The figure shows three views and two pictorial views of one solid part (mm, origin at its lowest corner). Answer the questions. A direction names the side the tool comes from. Coordinates: 2 decimals unless noted, no trailing zeros. Loops run counter-clockwise (first coordinate to the right, second up) from the corner with the lowest first, then second, coordinate; pieces in that order, holes last. Notation, with made-up numbers: (7.25, 82) -> (17.25, 82) arc R30 cw to (17.25, 110) -> close; hole circle Ø1 at (38, 68). An arc over 180 degrees is marked (long way). Answer in a Markdown table with one row per item.
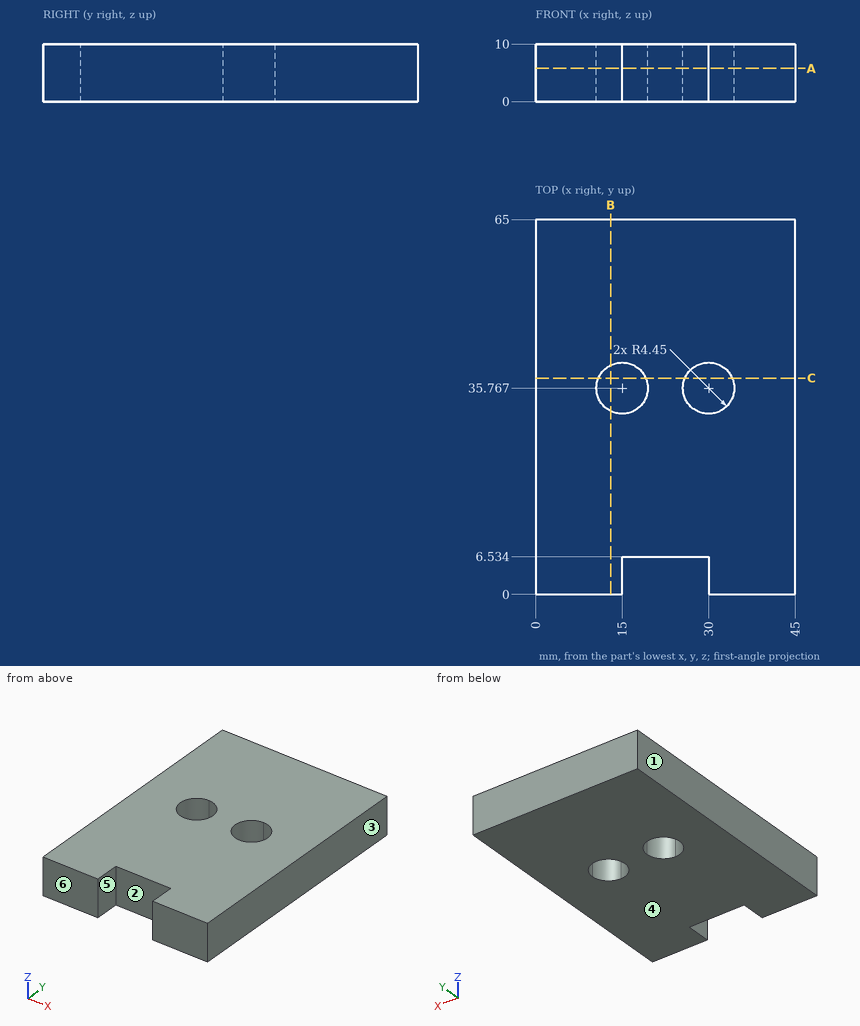
Item 1: A cutting plane is placed at A-A, the plane z = 5.75. Determine the outline of the cut face in (x, y), plus the area to 3 significant figures.
Findings below:
| item | result |
|---|---|
| outline | (0, 0) -> (15, 0) -> (15, 6.53) -> (30, 6.53) -> (30, 0) -> (45, 0) -> (45, 65) -> (0, 65) -> close; hole (15, 40.22) arc R4.45 ccw (long way) to (19.45, 35.77) arc R4.45 ccw to start; hole (30, 40.22) arc R4.45 ccw (long way) to (34.45, 35.77) arc R4.45 ccw to start |
| area | 2,700 mm2 |
Item 2: A tool of negligible diameter and unlimited length cuts with its end or side. For the marked faces 5 and 6, from which of +Z, -Z, +X, -X, +Y, -Y can it reach the whole face along a straight path? Write none if from no direction.
Findings below:
| item | result |
|---|---|
| face 5 | +Z, -Z, -Y |
| face 6 | +Z, -Z, +X, -X, -Y |
Item 3: Determine the mould class of the marked faces 1, 2, 3 and 4 for opening direction X: +X half, -X half, draft (parallel to the pull), parting line (faces both ways), or undercut.
Findings below:
| item | result |
|---|---|
| face 1 | -X half |
| face 2 | undercut |
| face 3 | +X half |
| face 4 | draft |
Item 4: A cutting plane is placed at B-B, the plane x = 13. Determine the outline of the cut face in (y, z).
Findings below:
| item | result |
|---|---|
| outline | (0, 0) -> (31.79, 0) -> (31.79, 10) -> (0, 10) -> close; (39.74, 0) -> (65, 0) -> (65, 10) -> (39.74, 10) -> close |
Item 5: Find the intervals of material crossed by probe 1 along X at (y, z) = (34, 0.5) (1 decimal); probe 2 along X at (y, z) = (6, 6); probe 3 along Y at (x, z) = (19, 5.25) (1 decimal), in increasing order.
Findings below:
| item | result |
|---|---|
| probe 1 | x = 0 to 10.9, 19.1 to 25.9, 34.1 to 45 |
| probe 2 | x = 0 to 15, 30 to 45 |
| probe 3 | y = 6.5 to 33.8, 37.7 to 65 |
Item 6: A cutting plane is placed at C-C, the plane y = 37.5. Determine the outline of the cut face in (x, z), plus the area to 3 significant figures.
Findings below:
| item | result |
|---|---|
| outline | (0, 0) -> (10.9, 0) -> (10.9, 10) -> (0, 10) -> close; (19.1, 0) -> (25.9, 0) -> (25.9, 10) -> (19.1, 10) -> close; (34.1, 0) -> (45, 0) -> (45, 10) -> (34.1, 10) -> close |
| area | 286 mm2 |
Item 7: Flat-ended cylindrical pins translate along their axes: pin 1 Ø3 at (x, z) = (24, 3.5) entering from -Y; pin 2 Ø1 at (x, y) = (12, 33.5) entering from +Z. Find the tip coordinate at first contact, or state that the pin passes through.
Findings below:
| item | result |
|---|---|
| pin 1 | stops at y = 6.53 |
| pin 2 | passes through |
